Verification items for the finished model (mm, model axes). Face numbers are marked on the shaded views. A direction names the side the tool comes from. Round coordinates to 2 decimals unless told otherwise and drop trailing zeros. Write each loop counter-clockwise with the first axis right and the second up, starting at its lowest first coordinate (ties: lowest second). Pieces come first, ordered by that corner, then holes. Notation, with made-up numbers: (59, 64) - (78, 64) arc R24 ccw to (78, 100) - close; hole circle Ø8 at (77, -40). An arc over 180 degrees is marked (long way). Answer as a JSON object with one key per item and string values. Group by question number.
1) Mould release check, pull along X, two halves, no side actions. Record for the marked faces 5, 6, 7 and 8: +X half, -X half, draft (parallel to the pull), parting line (faces both ways), or undercut.
2) Section check C-C (y = 10.25). Enter the section's corners in (x, z).
3) Section check D-D (y = 3.75). Enter the section's corners in (x, z).
4) Section check B-B (x = -8). Enter the section's corners in (y, z), then the cut area to 3 significant figures.
5) Section check A-A (z = -10.5). Enter the section's corners in (x, y).
6) Thickness scan on line 1 (Y direction, x = -9, z = -14); line 2 (X direction, y = 4, z = 1); line 3 (Y direction, x = 15, z = 14). Record the ranges inside material, lowest first.
7) Go/stop test with flat-tipped pins: pin 1 Ø10 at (y, z) = (11, 8.5) entering from +X; pin 2 Ø0.6 at (y, z) = (29, 18) entering from +X; pin 3 Ø11.5 at (x, z) = (6, 0) entering from +Y; pin 4 Ø8 at (y, z) = (8.5, 2) entering from -X. Record where each tip stops, or that it passes through.
8) Set-up check for the marked faces 1, 2, 3 and 4: record each of +Z, -Z, +X, -X, +Y, -Y from which the full face is reachable in a straight line by a thin tool's end or side.
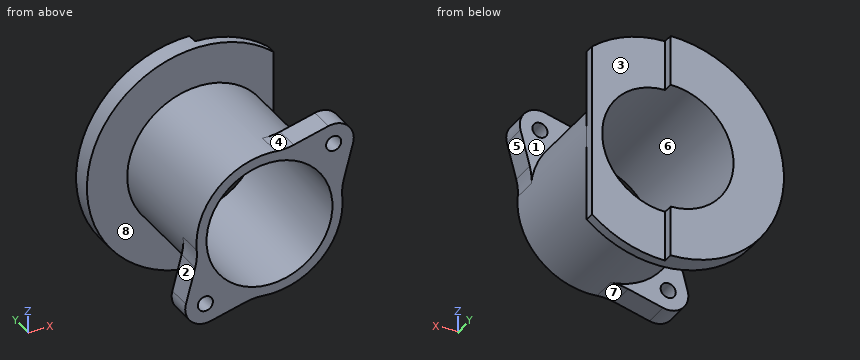
```python
from build123d import *

# Parameters (mm, degrees)
SKETCH_2_R          = 14.5
SKETCH_2_R_2        = 12.5
EXTRUDE_1_DEPTH     = 25.5
SKETCH_3_R          = 22.5
SKETCH_3_R_2        = 12.5
EXTRUDE_2_DEPTH     = 2
EXTRUDE_3_DEPTH     = 2
CUT_EXTRUDE_1_DEPTH = 10
SKETCH_7_R          = 1.500000000000006
SKETCH_7_R_2        = 14.5
SKETCH_7_R_3        = 12.5
SKETCH_7_R_4        = 1.499999999999986
EXTRUDE_4_DEPTH     = 5
FILLET_1_R          = 10


with BuildPart() as part:
    # 草圖2 → 填料-伸長1 (new body)
    with BuildSketch(Plane(origin=(0, 0, 0), x_dir=(1, 0, 0), z_dir=(0, 1, 0))):
        with Locations(Location((0, 0, 0), (0, 0, 270))):
            Circle(SKETCH_2_R)
        with Locations(Location((0, 0, 0), (0, 0, 270))):
            Circle(SKETCH_2_R_2, mode=Mode.SUBTRACT)
    extrude(amount=EXTRUDE_1_DEPTH)

    # 草圖3 → 填料-伸長2 (add)
    with BuildSketch(Plane(origin=(0, 25.5, 0), x_dir=(1, 0, 0), z_dir=(0, 1, 0))):
        with Locations(Location((0, 0, 0), (0, 0, 270))):
            Circle(SKETCH_3_R)
        with Locations(Location((0, 0, 0), (0, 0, 270))):
            Circle(SKETCH_3_R_2, mode=Mode.SUBTRACT)
    extrude(amount=EXTRUDE_2_DEPTH)

    # 草圖4 → 填料-伸長3 (add)
    with BuildSketch(Plane(origin=(0, 27.499999999999996, 0), x_dir=(1, 0, 0), z_dir=(0, 1, 0))):
        with BuildLine():
            Line((0, 22.500000000000004), (4.29e-15, 12.5))
            ThreePointArc((4.29e-15, 12.5), (-12.5, 1.53e-15), (4.29e-15, -12.5))
            Line((4.29e-15, -12.5), (0, -22.500000000000004))
            ThreePointArc((0, -22.500000000000004), (-22.500000000000004, 2.76e-15), (0, 22.500000000000004))
        make_face()
    extrude(amount=EXTRUDE_3_DEPTH)

    # 草圖6 → 除料-伸長1 (cut)
    with BuildSketch(Plane.XZ.offset(-25.5)):
        Polygon((14.499999999999996, 29.395789513712703), (53.33899904059902, 29.395789513712703), (53.33899904059903, -31.21012107711215), (14.500000000000004, -31.21012107711215), align=None)
    extrude(amount=-CUT_EXTRUDE_1_DEPTH, mode=Mode.SUBTRACT)

    # 草圖7 → 填料-伸長4 (add)
    # profile 1 of 3: a face of its own
    with BuildSketch(Plane.XZ):
        with BuildLine():
            ThreePointArc((-16.59162536651419, -11.692645880947747), (-15.556349186104121, -15.556349186104029), (-11.692645880947847, -16.591625366514123))
            Line((-11.692645880947847, -16.591625366514123), (-2.839123359878414, -14.21933115682284))
            ThreePointArc((-2.8391233598784202, -14.219331156822836), (-10.253048327204969, -10.25304832720491), (-14.219331156822854, -2.8391233598783336))
            Line((-14.219331156822806, -2.8391233598783234), (-16.59162536651419, -11.692645880947747))
        make_face()
        with Locations(Location((-12.727922061357921, -12.72792206135785, 0), (0, 0, 270))):
            Circle(SKETCH_7_R, mode=Mode.SUBTRACT)
    # profile 2 of 3: a face of its own
    with BuildSketch(Plane.XZ):
        with Locations(Location((0, 0, 0), (0, 0, 258.708444725))):
            Circle(SKETCH_7_R_2)
        with Locations(Location((0, 0, 0), (0, 0, 90))):
            Circle(SKETCH_7_R_3, mode=Mode.SUBTRACT)
    # profile 3 of 3: a face of its own
    with BuildSketch(Plane.XZ):
        with BuildLine():
            Line((11.692645880947822, 16.591625366514), (2.839123359878405, 14.21933115682271))
            ThreePointArc((2.8391233598784344, 14.219331156822834), (10.253048327205017, 10.25304832720486), (14.219331156822877, 2.8391233598782186))
            Line((14.219331156822797, 2.8391233598782026), (16.591625366514172, 11.692645880947598))
            ThreePointArc((16.591625366514172, 11.692645880947598), (15.556349186104118, 15.556349186103905), (11.692645880947822, 16.591625366514))
        make_face()
        with Locations(Location((12.727922061357914, 12.72792206135772, 0), (0, 0, 270))):
            Circle(SKETCH_7_R_4, mode=Mode.SUBTRACT)
    extrude(amount=-EXTRUDE_4_DEPTH)

    # 圓角1
    # the kernel refuses this fillet: 10 mm, written as the material it adds along each edge
    with BuildSketch(Plane(origin=(-14.21933115682283, 0, -2.8391233598783296), x_dir=(-0.14301440720376446, 0, 0.9897206067027986), z_dir=(0, 1, 0))) as fillet_1_piece_1:
        with BuildLine():
            CenterArc((2.0881667201812895, -9.98565558877935), FILLET_1_R, 93.06924050881132, 20.153074257108685)
            Line((-1.8548317977652202, -0.7958371636160083), (0, 0))
            ThreePointArc((0, 0), (0.7763696780160548, -0.02079939626993994), (1.5527393560321237, -3e-17))
        make_face()
    extrude(amount=5)
    with BuildSketch(Plane(origin=(2.83912335987842, 0, 14.219331156822772), x_dir=(-0.9897206067027934, 0, 0.1430144072038011), z_dir=(0, 1, 0))) as fillet_1_piece_2:
        with BuildLine():
            CenterArc((2.0881667201813614, 9.98565558877934), FILLET_1_R, 246.7776852340785, 20.153074257108983)
            Line((-1.854831797765394, 0.7958371636161028), (0, 0))
            ThreePointArc((0, 0), (0.7763696780159942, 0.02079939626995778), (1.552739356031987, -2e-17))
        make_face()
    extrude(amount=5)
    with BuildSketch(Plane(origin=(14.219331156822836, 0, 2.839123359878211), x_dir=(0.14301440720376882, 0, -0.989720606702798), z_dir=(0, 1, 0))) as fillet_1_piece_3:
        with BuildLine():
            CenterArc((2.088166720181273, -9.985655588779348), FILLET_1_R, 93.06924050881172, 20.1530742571085)
            Line((-1.8548317977652724, -0.795837163616021), (0, 0))
            ThreePointArc((0, 0), (0.7763696780160197, -0.02079939626995059), (1.5527393560320395, 2e-17))
        make_face()
    extrude(amount=5)
    with BuildSketch(Plane(origin=(-2.8391233598784176, 0, -14.21933115682284), x_dir=(0.9897206067028005, 0, -0.1430144072037512), z_dir=(0, 1, 0))) as fillet_1_piece_4:
        with BuildLine():
            CenterArc((2.088166720181194, 9.985655588779359), FILLET_1_R, 246.7776852340814, 20.153074257108187)
            Line((-1.8548317977650892, 0.7958371636159217), (0, 0))
            ThreePointArc((0, 0), (0.7763696780160907, 0.02079939626993076), (1.552739356032181, -2e-17))
        make_face()
    extrude(amount=5)


solid = part.part
```
Returned:
{
 "1": {"face 5": "+X half", "face 6": "undercut", "face 7": "undercut", "face 8": "draft"},
 "2": {"outline": "circle Ø29 at (0, 0); hole circle Ø25 at (0, 0)"},
 "3": {"outline": "(-16.59, -11.69) arc R4 ccw to (-11.69, -16.59) - (-4.79, -14.74) arc R10 cw to (-1.3, -14.44) arc R14.5 ccw to (14.44, 1.3) arc R10 cw to (14.74, 4.79) - (16.59, 11.69) arc R4 ccw to (11.69, 16.59) - (4.79, 14.74) arc R10 cw to (1.3, 14.44) arc R14.5 ccw to (-14.44, -1.3) arc R10 cw to (-14.74, -4.79) - close; hole circle Ø3 at (-12.73, -12.73); hole circle Ø25 at (0, 0); hole circle Ø3 at (12.73, 12.73)"},
 "4": {"outline": "(0, -15.6) - (5, -15.6) - (5, -12.09) - (25.5, -12.09) - (25.5, -21.03) - (29.5, -21.03) - (29.5, -9.6) - (0, -9.6) - close; (0, 9.6) - (29.5, 9.6) - (29.5, 21.03) - (25.5, 21.03) - (25.5, 12.09) - (0, 12.09) - close", "area": "236 mm2"},
 "5": {"outline": "(-19.9, 25.5) - (-10, 25.5) - (-10, 5) - (-16.27, 5) - (-16.27, 0) - (-6.78, 0) - (-6.78, 29.5) - (-19.9, 29.5) - close; (6.78, 0) - (10, 0) - (10, 25.5) - (14.5, 25.5) - (14.5, 27.5) - (6.78, 27.5) - close"},
 "6": {"line 1": "0 to 5, 25.5 to 29.5", "line 2": "-14.47 to -12.46, 12.46 to 14.47", "line 3": "0 to 5"},
 "7": {"pin 1": "x = 14.07", "pin 2": "x = 0", "pin 3": "through", "pin 4": "x = -14.5"},
 "8": {"face 1": "+Z, +X", "face 2": "+Z, -X, -Y", "face 3": "+Z, -Z, +X, +Y", "face 4": "+Z, -Y"}
}
